Could you check a few things on this model? Use its own coordinates, in mm. Round coordinates to 2 decimals unless told otherwise and drop trailing zeros. Write each loop counter-clockwise with the first axis right and the second up, starting at its lowest first coordinate (ties: lowest second). Pieces come first, ordered by that corner, then holes. Notation, with made-up numbers: (66.5, 59.5) -> (118.5, 59.5) arc R4 ccw to (118.5, 65.5) -> close; hole circle Ø11 at (57, 19). An arc over 180 degrees is marked (long way). One line per question, with ' | ' between items. Start each with the question number.
1. Imagine slicing it at D-D, the plane y = -0.1. List the corners of the cut face in (x, z) for me (3 decimals), and give its area (3 significant figures).
2. For pin 1 Ø3 at (y, z) = (10.5, 3.5) entering from +X (3 decimals); pin 2 Ø3 at (x, z) = (-171.5, 4) entering from -Y; pin 3 Ø3 at (x, z) = (-172.5, 1.5) entering from +Y, each with a flat end and sliding along its axis, tell me the tip position at first contact or that it passes through.
3. Imagine slicing it at B-B, the plane y = 27. List the corners of the cut face in (x, z) for me (3 decimals), and give its area (3 significant figures).
4. Imagine slicing it at A-A, the plane x = 50.8. List the corners of the cut face in (y, z) for me, and give its area (3 significant figures).
5. Imagine slicing it at C-C, the plane z = 2. List the corners of the cut face in (x, y) for me (3 decimals).
6. If I drill on line 1 along Y through (x, z) = (-50.8, 2); line 2 along X through (y, z) = (11, 3.5) (3 decimals); line 3 along X through (y, z) = (26, 5.75) (3 decimals), over which ranges is the centre line in solid material (lowest first)? Write a range as [from, to].
from build123d import *

# Parameters (mm, degrees)
BOSS_EXTRUDE1_DEPTH      = 6.35
F_0_257_DIAMETER_HOLE1_D = 6.5278


with BuildPart() as part:
    # Sketch1 → Boss-Extrude1 (new body)
    with BuildSketch(Plane.XY):
        Polygon((-168.275, -6.35), (-168.275, -12.7), (-142.875, -12.7), (-9.525, -12.7), (9.525, -12.7), (142.875, -12.7), (168.275, -12.7), (168.275, -6.35), (174.625, -6.35), (174.625, 6.15), (168.275, 6.15), (168.275, 12.7), (168.275, 19.25), (174.625, 19.25), (174.625, 31.75), (168.275, 31.75), (168.275, 38.1), (155.575, 38.1), (142.875, 12.7), (9.525, 12.7), (-9.525, 12.7), (-142.875, 12.7), (-155.575, 38.1), (-168.275, 38.1), (-168.275, 31.75), (-174.625, 31.75), (-174.625, 19.25), (-168.275, 19.25), (-168.275, 12.7), (-168.275, 6.15), (-174.625, 6.15), (-174.625, -6.35), align=None)
    extrude(amount=BOSS_EXTRUDE1_DEPTH)

    # F (0.257) Diameter Hole1 (through all)
    with Locations(Plane.XY.offset(6.35)):
        with Locations((-50.8, -0.1), (50.8, -0.1)):
            Hole(F_0_257_DIAMETER_HOLE1_D / 2)


solid = part.part
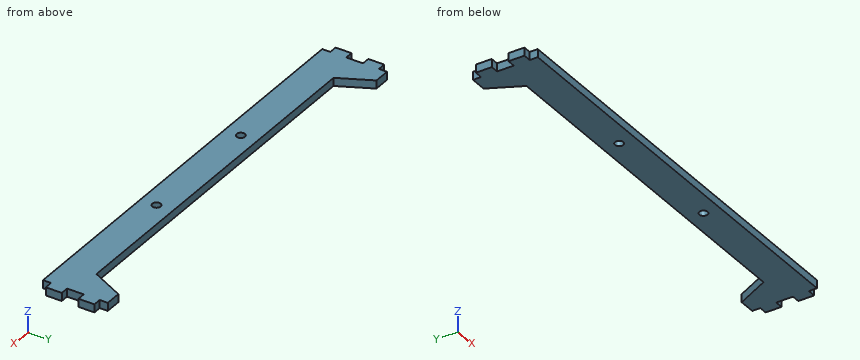
Geometry results:
1) outline: (-174.625, 0) -> (-54.064, 0) -> (-54.064, 6.35) -> (-174.625, 6.35) -> close; (-47.536, 0) -> (47.536, 0) -> (47.536, 6.35) -> (-47.536, 6.35) -> close; (54.064, 0) -> (174.625, 0) -> (174.625, 6.35) -> (54.064, 6.35) -> close | area: 2,130 mm2
2) pin 1: stops at x = 168.275 | pin 2: stops at y = -6.35 | pin 3: stops at y = 31.75
3) outline: (-174.625, 0) -> (-150.025, 0) -> (-150.025, 6.35) -> (-174.625, 6.35) -> close; (150.025, 0) -> (174.625, 0) -> (174.625, 6.35) -> (150.025, 6.35) -> close | area: 312 mm2
4) outline: (-12.7, 0) -> (-3.36, 0) -> (-3.36, 6.35) -> (-12.7, 6.35) -> close; (3.16, 0) -> (12.7, 0) -> (12.7, 6.35) -> (3.16, 6.35) -> close | area: 120 mm2
5) outline: (-174.625, -6.35) -> (-168.275, -6.35) -> (-168.275, -12.7) -> (168.275, -12.7) -> (168.275, -6.35) -> (174.625, -6.35) -> (174.625, 6.15) -> (168.275, 6.15) -> (168.275, 19.25) -> (174.625, 19.25) -> (174.625, 31.75) -> (168.275, 31.75) -> (168.275, 38.1) -> (155.575, 38.1) -> (142.875, 12.7) -> (-142.875, 12.7) -> (-155.575, 38.1) -> (-168.275, 38.1) -> (-168.275, 31.75) -> (-174.625, 31.75) -> (-174.625, 19.25) -> (-168.275, 19.25) -> (-168.275, 6.15) -> (-174.625, 6.15) -> close; hole circle Ø6.528 at (-50.8, -0.1); hole circle Ø6.528 at (50.8, -0.1)
6) line 1: y = [-12.7, -3.36], [3.16, 12.7] | line 2: x = [-168.275, 168.275] | line 3: x = [-174.625, -149.525], [149.525, 174.625]
